from build123d import *

# Parameters (mm, degrees)
F2_R          = 31.75
F3_DEPTH      = 211.2122471454
F3_DEPTH_BACK = 288.1372322342


with BuildPart() as f1:
    # F0 (on Top) → F1 (revolve)
    with BuildSketch(Plane.XY):
        Polygon((207.1876852567, 0), (-288.1362322342, -4.5483284574), (-284.1126703454, -182.3027966142), (-265.0675487572, -181.8717006976), (-267.9034604739, -100.6019149123), (190.1752766148, -90.2330720489), (192.1661255572, -178.1855640735), (211.2112471454, -177.7544681569), align=None)
    revolve(axis=Axis((-40.4742734887, -2.2741642287, 0), (0.9999578432, 0.0091821464, 0)))

    # F2 (on Right) → F3 (cut, two sides)
    with BuildSketch(Plane.YZ) as f3_sk:
        Circle(F2_R)
    extrude(amount=F3_DEPTH, mode=Mode.SUBTRACT)
    extrude(f3_sk.sketch, amount=-F3_DEPTH_BACK, mode=Mode.SUBTRACT)


solid = f1.part
For this review, take the finished solid that the model builds, in its own axes (mm). A direction names the side the tool comes from. Give positions to 0.01 mm unless a question says otherwise; leave off trailing zeros.
Item 1: Tool access review of faces 3 (the conical face through (189.23, 20.55, 93.3)), 4 (the conical face through (207.664, 5.061, -38.508)): name each direction out of +Z, -Z, +X, -X, +Y, -Y from which nothing blocks a thin tool from reaching the whole face with its end or side.
Item 2: Draft analysis for pull direction Y (two halves, no side actions). For faces 1 (the conical face through (-269.605, 95.712, -4.405)), 2 (the conical face through (202.09, 23.11, -176.37)), state which applies: +Y half, -Y half, draft (parallel to the pull), parting line (faces both ways), or undercut.
Item 3: Insertion check: pin 1 (5 mm diameter, centred on y = 103, z = -4, fed in from +X); pin 2 (1 mm diameter, centred on x = -149, y = 77, fed in from +Z); pin 3 (12 mm diameter, centred on y = 48, z = -23, fed in from -X). Each pin has a flat end and moves straight along its axis. Give the tip position at first contact, or say it passes through.
Item 4: For line 1 along Z through (x, y) = (-65, 0); line 2 along Z through (x, y) = (-51, 0); line 3 along Y through (x, z) = (-10, 0), list the stretches that pass through material, from the lowest coordinate up.
Calculated:
1. face 3: none
1. face 4: +X
2. face 1: undercut
2. face 2: parting line
3. pin 1: stops at x = 207.64
3. pin 2: stops at z = 50.88
3. pin 3: stops at x = -287.88
4. line 1: z = -93.46 to -31.75, 31.75 to 93.46
4. line 2: z = -93.28 to -31.75, 31.75 to 93.28
4. line 3: y = -94.76 to -31.75, 31.75 to 90.75
